Here's how the part is built. I have some questions about the finished solid (model axes, mm). A direction names the side the tool comes from. Give positions to 0.01 mm unless a question says otherwise; leave off trailing zeros. Loops run counter-clockwise (first coordinate to the right, second up) from the corner with the lowest first, then second, coordinate; pieces in that order, holes last. Notation, with made-up numbers: M 53.5,12 L 106.5,12 A30 ccw 106.5,40 Z; hole C 37.5,38 d10. An arc over 180 degrees is marked long. Answer as CSV lines item,"result". Start each with the question number.
Item 1: I want a section at A-A on y = 0. List the corners of the cut face in (x, z) for me, plus the area to 3 significant figures.
Item 2: Will these pins go through, and if not, where does the flat tip stop? P1, Ø4, axis at x = 0, z = 2.25, coming from the -Y side; P2, Ø1.5, axis at x = 0, z = -2.5, coming from the -Y side; P3, Ø3, axis at y = 6.5, z = -2, coming from the -X side; P4, Ø3, axis at x = 4.68, y = -8.1, coming from the +Z side.
Item 3: I want a section at B-B on z = -2.5. List the corners of the cut face in (x, y) for me (3 decimals).
Item 4: For faces 1 (the cylindrical face through (1.25, -4.34, 2.3)), 2 (the flat face through (5.5, 3, 0)), which set-ups out of +Z, -Z, +X, -X, +Y, -Y let a thin tool reach every point of the face, with its end or its side?
Item 5: I want a section at C-C on x = 5.25. List the corners of the cut face in (y, z) for me.
Item 6: If we mould it in two halves opening along X, with no side actions, what happens to faces 3 (the cylindrical face through (-2.75, -12.4, -2.46)), 4 (the cylindrical face through (0.16, 7.64, -3.74)), 5 (the flat face through (-3, -1, 4.5))? For each: released by +X, released by -X, zero draft, split by the parting line, or undercut.
Item 7: I want a section at D-D on z = 2.25. List the corners of the cut face in (x, y) for me.
Item 8: If I drill on line 1 along Z through (x, y) = (0, -4.5); line 2 along Z through (x, y) = (0, -10); line 3 along X through (y, z) = (-8, -2.5), over which ranges is the centre line in solid material (lowest first)? Write a range as from..to.
Autodesk Inventor part; units mm, degrees
ref_plane "YZ Plane" through (0, 0, 0) normal (1, 0, 0) x (0, 1, 0)
ref_plane "XZ Plane" through (0, 0, 0) normal (0, 1, 0) x (-1, 0, 0)
ref_plane "XY Plane" through (0, 0, 0) normal (0, 0, 1) x (1, 0, 0)
sketch "Base" plane through (0, 0, 0) normal (0, 0, 1) x (1, 0, 0)
  circle A0 centre (0, 0) radius 3
  circle A1 centre (0, 0) radius 6
  circle A2 centre (0, 0) radius 12.7
  circle A3 centre (0, 0) radius 9.35 construction
  line L0 (0, 6) -> (0, 12.7) construction
  line L1 (0, -17.78) -> (0, 17.78) construction
  circle A4 centre (-9.35, 0) radius 1.25
  line L2 (-17.78, 0) -> (17.78, 0) construction
  circle A5 centre (-4.675, -8.0973) radius 1.25
  circle A6 centre (4.675, -8.0973) radius 1.25
  circle A7 centre (9.35, 0) radius 1.25
  circle A8 centre (4.675, 8.0973) radius 1.25
  circle A9 centre (-4.675, 8.0973) radius 1.25
  point P0 (0, 9.35)
  dimension "d1" = 12
  dimension "d2" = 25.4
  dimension "d0" = 6
  dimension "d3" = 2.5
  dimension "d6" = 360
extrude "BaseFeature" add sketch "Base" against normal blind 5 contours A1 | A2
extrude "FlangeFeature" add sketch "Base" along normal blind 4.5 contours A1
sketch "FixatingHoles" plane through (0, 0, 0) normal (0, 1, 0) x (-1, 0, 0)
  line L0 (-3, 4.5) -> (3, 4.5) construction
  line L1 (0, 4.5) -> (0, 0) construction
  line L2 (12.7, 0) -> (-12.7, 0)
  line L3 (3, -5) -> (-3, -5) construction
  line L4 (0, -5) -> (0, 0) construction
  circle A0 centre (0, 2.25) radius 1.25
  circle A1 centre (0, -2.5) radius 1.25
  dimension "d12" = 2.5
  dimension "d13" = 2.5
extrude "FixatingHolesFeature" cut sketch "FixatingHoles" along normal through all both and the other way through all
properties part number "PololuHub1994"
Result:
1,outline,"M -12.7,-5 L -10.6,-5 L -10.6,0 L -12.7,0 Z; M -8.1,-5 L -3,-5 L -3,4.5 L -6,4.5 L -6,0 L -8.1,0 Z; M 3,-5 L 8.1,-5 L 8.1,0 L 6,0 L 6,4.5 L 3,4.5 Z; M 10.6,-5 L 12.7,-5 L 12.7,0 L 10.6,0 Z"
1,area,"99.0 mm^2"
2,P1,"y = -6"
2,P2,"through"
2,P3,"x = -11.67"
2,P4,"z = 0"
3,outline,"M -1.25,-12.638 L -1.25,-2.727 A3 cw -1.25,2.727 L -1.25,12.638 A12.7 ccw Z; M 1.25,-12.638 A12.7 ccw 1.25,12.638 L 1.25,2.727 A3 cw 1.25,-2.727 Z; hole C -9.35,0 d2.5; hole C -4.675,-8.097 d2.5; hole C -4.675,8.097 d2.5; hole C 4.675,-8.097 d2.5; hole C 4.675,8.097 d2.5; hole C 9.35,0 d2.5"
4,face 1,"+Y, -Y"
4,face 2,"+Z"
5,outline,"M -11.56,-5 L -9.21,-5 L -9.21,0 L -11.56,0 Z; M -6.99,-5 L 6.99,-5 L 6.99,0 L 2.9,0 L 2.9,4.5 L -2.9,4.5 L -2.9,0 L -6.99,0 Z; M 9.21,-5 L 11.56,-5 L 11.56,0 L 9.21,0 Z"
6,face 3,"split by the parting line"
6,face 4,"undercut"
6,face 5,"zero draft"
7,outline,"M -1.25,-5.87 L -1.25,-2.73 A3 cw -1.25,2.73 L -1.25,5.87 A6 ccw Z; M 1.25,-5.87 A6 ccw 1.25,5.87 L 1.25,2.73 A3 cw 1.25,-2.73 Z"
8,line 1,"-5..-3.75, -1.25..1, 3.5..4.5"
8,line 2,"-5..-3.75, -1.25..0"
8,line 3,"-9.86..-5.92, -3.43..-1.25, 1.25..3.43, 5.92..9.86"
